The model under review builds one solid part; all positions refer to its coordinate system, in mm. A direction names the side the tool comes from. Give positions to 0.01 mm unless a question says otherwise; leave off trailing zeros. Write each loop counter-clockwise with the first axis right and the second up, starting at its lowest first coordinate (ties: lowest second). Pieces come first, ordered by that corner, then holes. Notation, with made-up numbers: M 13.25,77.5 L 70.25,77.5 A33 ccw 70.25,106.5 Z; hole C 57.5,44.5 d6. An arc over 180 degrees is marked long. Write item = value, one per line. Start each with the question number.
```python
from build123d import *

# Parameters (mm, degrees)
CUT_EXTRUDE1_DEPTH = 95.25


with BuildPart() as part:
    # Sketch1 → Revolve1 (revolve)
    with BuildSketch(Plane.XY, mode=Mode.PRIVATE) as revolve1_sk:
        with BuildLine():
            Line((0, 0), (0, 8.58901))
            Line((0, 8.58901), (0.93599, 9.525))
            Line((0.93599, 9.525), (9.344692072, 9.525))
            Line((9.344692072, 9.525), (10.348204118, 8.708440423))
            ThreePointArc((10.348204118, 8.708440423), (10.611556372, 8.560342712), (10.9093, 8.509))
            Line((10.9093, 8.509), (12.4714, 8.509))
            ThreePointArc((12.4714, 8.509), (13.100017928, 8.769382072), (13.3604, 9.398))
            Line((13.3604, 9.398), (13.3604, 9.49325))
            Line((13.3604, 9.49325), (15.748, 9.49325))
            Line((15.748, 9.49325), (15.748, 0))
            Line((15.748, 0), (0, 0))
        make_face()
    revolve(revolve1_sk.sketch.rotate(Axis((15.748, 0, 0), (-1, 0, 0)), 270), axis=Axis((15.748, 0, 0), (-1, 0, 0)))

    # Sketch2 → Revolve2 (revolve)
    with BuildSketch(Plane.XY, mode=Mode.PRIVATE) as revolve2_sk:
        Polygon((15.748, 0), (15.748, 19.00555), (16.51, 19.76755), (41.2115, 19.76755), (41.2115, 18.18005), (42.2275, 18.18005), (43.2435, 19.19605), (46.863, 19.19605), (47.625, 18.43405), (47.625, 0), align=None)
    revolve(revolve2_sk.sketch.rotate(Axis((47.625, 0, 0), (-1, 0, 0)), 270), axis=Axis((47.625, 0, 0), (-1, 0, 0)))

    # Sketch3 → Cut-Revolve1 (revolve, cut)
    with BuildSketch(Plane(origin=(0, 0, 0), x_dir=(1, 0, 0), z_dir=(0, 1, 0)), mode=Mode.PRIVATE) as cut_revolve1_sk:
        Polygon((31.75, 0), (34.925, 0), (34.925, -8.330850926), (36.256425852, -9.09955), (36.569651116, -19.132537191), (37.204663925, -19.76755), (31.75, -19.76755), align=None)
    revolve(cut_revolve1_sk.sketch.rotate(Axis((31.75, 0, 19.76755), (0, 0, -1)), 180), axis=Axis((31.75, 0, 19.76755), (0, 0, -1)), mode=Mode.SUBTRACT)

    # Sketch4 → Revolve3 (revolve)
    with BuildSketch(Plane.XY, mode=Mode.PRIVATE) as revolve3_sk:
        with BuildLine():
            Line((41.2115, 17.92605), (42.2275, 17.92605))
            Line((42.2275, 17.92605), (42.2275, 18.18005))
            Line((42.2275, 18.18005), (41.7195, 18.18005))
            Line((41.7195, 18.18005), (41.344882072, 18.554667928))
            ThreePointArc((41.344882072, 18.554667928), (41.307684633, 18.64447049), (41.344882072, 18.734273051))
            Line((41.344882072, 18.734273051), (42.293990825, 19.683381804))
            Line((42.293990825, 19.683381804), (42.293990825, 19.76755))
            Line((42.293990825, 19.76755), (42.090790825, 19.76755))
            Line((42.090790825, 19.76755), (41.2115, 18.888259175))
            Line((41.2115, 18.888259175), (41.2115, 17.92605))
        make_face()
    revolve(revolve3_sk.sketch.rotate(Axis((42.2275, 0, 0), (-1, 0, 0)), 270), axis=Axis((42.2275, 0, 0), (-1, 0, 0)))

    # Sketch5 → Cut-Extrude1 (cut)
    with BuildSketch(Plane(origin=(0, 0, 0), x_dir=(0, 0, -1), z_dir=(1, 0, 0))):
        with BuildLine():
            Line((-5.969, 3.683), (-5.969, -3.683))
            ThreePointArc((-5.969, -3.683), (-5.299446102, -5.299446102), (-3.683, -5.969))
            Line((-3.683, -5.969), (3.683, -5.969))
            ThreePointArc((3.683, -5.969), (5.299446102, -5.299446102), (5.969, -3.683))
            Line((5.969, -3.683), (5.969, 3.683))
            ThreePointArc((5.969, 3.683), (5.299446102, 5.299446102), (3.683, 5.969))
            Line((3.683, 5.969), (-3.683, 5.969))
            ThreePointArc((-3.683, 5.969), (-5.299446102, 5.299446102), (-5.969, 3.683))
        make_face()
    extrude(amount=CUT_EXTRUDE1_DEPTH, mode=Mode.SUBTRACT)


solid = part.part
```
Item 1: The part is to be moulded in two halves that separate along Z. For faces 3 (the flat face through (23, -5.969, 0)), 4 (the cylindrical face through (23.5, -5.3, -5.3)), 5 (the conical face through (35.66, -3, 19.24)), 6 (the cylindrical face through (34.27, -1.93, 7.17)), say which applies: released by +Z, released by -Z, zero draft, split by the parting line, or undercut.
Item 2: We need section C-C, the plane x = 31.75. Write out the cut boundary in (y, z) (3 decimals).
Item 3: Clearance check with flat-ended pins moving along their axes: P1, Ø2, axis at x = 10.5, z = -4.5, coming from the +Y side (3 decimals); P2, Ø1.5, axis at x = 41.5, z = 13.5, coming from the -Y side; P3, Ø3, axis at x = 34.5, z = 15, coming from the -Y side. State where each tip first meets the part, or that it passes through.
Item 4: We need section A-A, the plane x = 20. Write out the cut boundary in (y, z).
Item 5: We need section B-B, the plane y = 0. Give the number of separate pieces and of enclosed holes in the cut face, and give its area (3 significant figures).
Item 6: For faces 1 (the flat face through (47.625, -8, 0)), 2 (the flat face through (23, 5.969, 0)), list the 3-axis set-ups (+Z, -Z, +X, -X, +Y, -Y) from which the entire face can be reached by the end or side of a thin tool; tool diameter is ignored.
Item 7: To check wall thickness, follow probe 1 along Z at (x, y) = (2, 0.5); probe 2 along X at (y, z) = (0, 7.1) (3 decimals); probe 3 along Z at (x, y) = (2.5, -1.5). State the ranges of each line that lie inside material, in increasing order. Write a range as [from, to].
Worked out:
q1.face_3 = undercut
q1.face_4 = undercut
q1.face_5 = released by +Z
q1.face_6 = zero draft
q2.outline = M -5.969,-3.683 L -5.969,3.683 A2.286 cw -3.683,5.969 L -3.175,5.969 L -3.175,8.331 L -4.506,9.1 L -4.82,19.133 L -4.85,19.163 A19.768 ccw long 4.85,19.163 L 4.82,19.133 L 4.506,9.1 L 3.175,8.331 L 3.175,5.969 L 3.683,5.969 A2.286 cw 5.969,3.683 L 5.969,-3.683 A2.286 cw 3.683,-5.969 L -3.683,-5.969 A2.286 cw Z
q3.P1 = 8.385
q3.P2 = -15.06
q3.P3 = -14.44
q4.outline = C 0,0 d39.54; hole M -5.97,-3.68 A2.29 ccw -3.68,-5.97 L 3.68,-5.97 A2.29 ccw 5.97,-3.68 L 5.97,3.68 A2.29 ccw 3.68,5.97 L -3.68,5.97 A2.29 ccw -5.97,3.68 Z
q5.separate_pieces = 3
q5.enclosed_holes = 0
q5.area = 852 mm²
q6.face_1 = +Z, -Z, +X, +Y, -Y
q6.face_2 = +X, -X
q7.probe_1 = [-9.51, -5.97], [5.97, 9.51]
q7.probe_2 = [0, 28.575], [34.925, 47.625]
q7.probe_3 = [-9.41, -5.97], [5.97, 9.41]
